Geometry: see drawing. Coordinates: mm, zero at the bounding-box minimum. A direction names the side the tool comes from. Round coordinates to 2 decimals unless told otherwise and drop trailing zeros. Write each loop counter-clockwise with the first axis right and the second up, starting at its lowest first coordinate (ties: lowest second). Pieces come first, ordered by that corner, then holes. Notation, with made-up numbers: M 42.5,74.25 L 80.5,74.25 A5 cw 80.5,82.25 Z; hole C 49.5,70 d3. An arc over 180 degrees is marked long. Use a Markdown table: item, result.
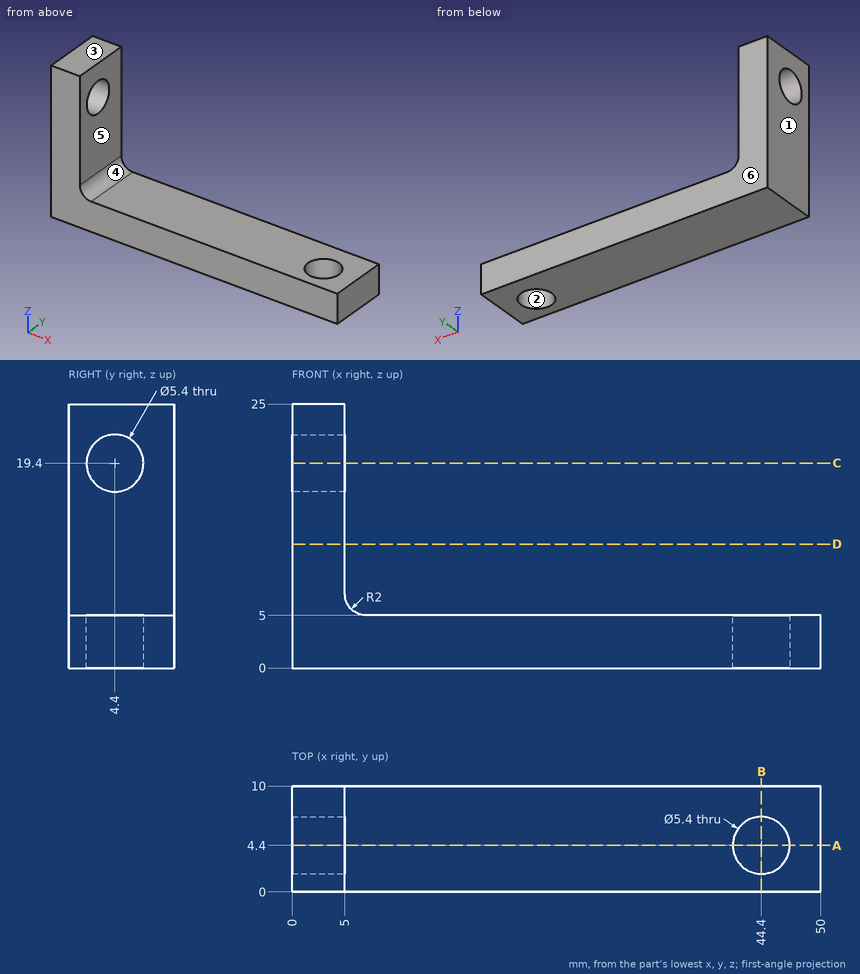
Q1. Line query: L1, parallel to Y at x = 44.4, z = 4; L2, parallel to X at y = 9.5, z = 11. Output: solid intervals per line, ascending.
Results are:
| item | result |
|---|---|
| L1 | 0 to 1.7, 7.1 to 10 |
| L2 | 0 to 5 |
Q2. First-contact query: pin 1 Ø2 at (y, z) = (7.5, 20) entering from +X; pin 2 Ø3 at (x, y) = (36.5, 3) entering from +Z; pin 3 Ø12 at (x, z) = (29, 13.5) entering from +Y. Flat tips, straight axial feed; report the tip coordinate or a pass-through.
Results are:
| item | result |
|---|---|
| pin 1 | x = 5 |
| pin 2 | z = 5 |
| pin 3 | through |
Q3. Section D-D on z = 11.75. Return loops of the section in (x, y), plus the area to 3 significant figures.
Results are:
| item | result |
|---|---|
| outline | M 0,0 L 5,0 L 5,10 L 0,10 Z |
| area | 50.0 mm^2 |
Q4. Mould query, pull axis X, two halves, no side actions, for the marked faces 1, 2, 3 and 4. Classes: +X half, -X half, draft (parallel to the pull), parting line (faces both ways), or undercut.
Results are:
| item | result |
|---|---|
| face 1 | -X half |
| face 2 | undercut |
| face 3 | draft |
| face 4 | +X half |
Q5. Section C-C on z = 19.4. Return loops of the section in (x, y), plus the area to 3 significant figures.
Results are:
| item | result |
|---|---|
| outline | M 0,0 L 5,0 L 5,1.7 L 0,1.7 Z; M 0,7.1 L 5,7.1 L 5,10 L 0,10 Z |
| area | 23.0 mm^2 |
Q6. Reachability of the marked faces 5 and 6 from +Z, -Z, +X, -X, +Y, -Y: full face, straight path, thin tool, end or side. Return the list, or none.
Results are:
| item | result |
|---|---|
| face 5 | +Z, +X, +Y, -Y |
| face 6 | +Z, -Z, +X, -X, +Y |
Q7. Section A-A on y = 4.4. Return loops of the section in (x, z).
Results are:
| item | result |
|---|---|
| outline | M 0,0 L 41.7,0 L 41.7,5 L 7,5 A2 cw 5,7 L 5,16.7 L 0,16.7 Z; M 0,22.1 L 5,22.1 L 5,25 L 0,25 Z; M 47.1,0 L 50,0 L 50,5 L 47.1,5 Z |
Q8. Section B-B on x = 44.4. Return loops of the section in (y, z).
Results are:
| item | result |
|---|---|
| outline | M 0,0 L 1.7,0 L 1.7,5 L 0,5 Z; M 7.1,0 L 10,0 L 10,5 L 7.1,5 Z |
